```python
from build123d import *

# Parameters (mm, degrees)
F0_W     = 9
F0_H     = 9
F0_H_2   = 441
F1_DEPTH = 18
F2_DEPTH = 9


# Not quite as in the source:
# - ends of sketch curves that miss each other by under 0.0002 mm in the source are joined


with BuildPart() as f1:
    # F0 (on Front) → F1 (new body)
    with BuildSketch(Plane.XZ):
        with Locations((-1095.5, 71.3756743552)):
            Rectangle(F0_W, F0_H)
        with BuildLine():
            Line((0, 66.8756743552), (-1091, 66.8756743552))
            Line((-1091, 66.8756743552), (-1091, -374.1243256448))
            Line((-1091, -374.1243256448), (-1055, -374.1243256448))
            ThreePointArc((-1055, -374.1243256448), (-1054.8038113281, -374.1191399972), (-1054.6076226562, -374.1243256448))
            Line((-1054.6076226562, -374.1243256448), (-973.3476458471, -374.1243256448))
            Line((-973.3476458471, -374.1243256448), (0, -374.1243256448))
            Line((0, -374.1243256448), (973.3476458471, -374.1243256448))
            Line((973.3476458471, -374.1243256448), (1054.6076226562, -374.1243256448))
            ThreePointArc((1054.6076226562, -374.1243256448), (1054.8038113281, -374.1191399972), (1055, -374.1243256448))
            Line((1055, -374.1243256448), (1091, -374.1243256448))
            Line((1091, -374.1243256448), (1091, -365.1243256448))
            Line((1091, -365.1243256448), (1091, -365.0378882885))
            Line((1091, -365.0378882885), (1091, 66.8756743552))
            Line((1091, 66.8756743552), (0, 66.8756743552))
        make_face()
        with BuildLine():
            Line((-1050, -320.6243256448), (-1050, 22.3756743552))
            ThreePointArc((-1050, 22.3756743552), (-1052.4748737342, 28.3505480894), (-1046.5, 25.8756743552))
            Line((-1046.5, 25.8756743552), (0, 25.8756743552))
            Line((0, 25.8756743552), (1046.5, 25.8756743552))
            ThreePointArc((1046.5, 25.8756743552), (1052.4748737342, 28.3505480894), (1050, 22.3756743552))
            Line((1050, 22.3756743552), (1050, -320.6243256448))
            ThreePointArc((1050, -320.6243256448), (1052.4748737342, -326.5991993789), (1046.5, -324.1243256448))
            Line((1046.5, -324.1243256448), (900, -324.1243256448))
            Line((900, -324.1243256448), (900, -338.6243256448))
            ThreePointArc((900, -338.6243256448), (902.4748737342, -344.5991993789), (896.5, -342.1243256448))
            Line((896.5, -342.1243256448), (753.5000238419, -342.1243256448))
            ThreePointArc((753.5000238419, -342.1243256448), (747.5251501077, -344.5991993789), (750.0000238419, -338.6243256448))
            Line((750.0000238419, -338.6243256448), (750.0000238419, -324.1243256448))
            Line((750.0000238419, -324.1243256448), (600.0000238419, -324.1243256448))
            Line((600.0000238419, -324.1243256448), (600, -338.6243256448))
            ThreePointArc((600, -338.6243256448), (602.4748737342, -344.5991993789), (596.5, -342.1243256448))
            Line((596.5, -342.1243256448), (453.5000238419, -342.1243256448))
            ThreePointArc((453.5000238419, -342.1243256448), (447.5251501077, -344.5991993789), (450.0000238419, -338.6243256448))
            Line((450.0000238419, -338.6243256448), (450.0000238419, -324.1243256448))
            Line((450.0000238419, -324.1243256448), (300.0000238419, -324.1243256448))
            Line((300.0000238419, -324.1243256448), (300, -338.6243256448))
            ThreePointArc((300, -338.6243256448), (302.4748737342, -344.5991993789), (296.5, -342.1243256448))
            Line((296.5, -342.1243256448), (153.5000238419, -342.1243256448))
            ThreePointArc((153.5000238419, -342.1243256448), (147.5251501077, -344.5991993789), (150.0000238419, -338.6243256448))
            Line((150.0000238419, -338.6243256448), (150.0000238419, -324.1243256448))
            Line((150.0000238419, -324.1243256448), (2.38419e-05, -324.1243256448))
            Line((2.38419e-05, -324.1243256448), (-150.0000238419, -324.1243256448))
            Line((-150.0000238419, -324.1243256448), (-150.0000238419, -338.6243256448))
            ThreePointArc((-150.0000238419, -338.6243256448), (-147.5251501077, -344.5991993789), (-153.5000238419, -342.1243256448))
            Line((-153.5000238419, -342.1243256448), (-296.5, -342.1243256448))
            ThreePointArc((-296.5, -342.1243256448), (-302.4748737342, -344.5991993789), (-300, -338.6243256448))
            Line((-300, -338.6243256448), (-300, -324.1243256448))
            Line((-300, -324.1243256448), (-450.0000238419, -324.1243256448))
            Line((-450.0000238419, -324.1243256448), (-450.0000238419, -338.6243256448))
            ThreePointArc((-450.0000238419, -338.6243256448), (-447.5251501077, -344.5991993789), (-453.5000238419, -342.1243256448))
            Line((-453.5000238419, -342.1243256448), (-596.5, -342.1243256448))
            ThreePointArc((-596.5, -342.1243256448), (-602.4748737342, -344.5991993789), (-600, -338.6243256448))
            Line((-600, -338.6243256448), (-600, -324.1243256448))
            Line((-600, -324.1243256448), (-750.0000238419, -324.1243256448))
            Line((-750.0000238419, -324.1243256448), (-750.0000238419, -338.6243256448))
            ThreePointArc((-750.0000238419, -338.6243256448), (-747.5251501077, -344.5991993789), (-753.5000238419, -342.1243256448))
            Line((-753.5000238419, -342.1243256448), (-896.5, -342.1243256448))
            ThreePointArc((-896.5, -342.1243256448), (-902.4748737342, -344.5991993789), (-900, -338.6243256448))
            Line((-900, -338.6243256448), (-900, -324.1243256448))
            Line((-900, -324.1243256448), (-1046.5, -324.1243256448))
            ThreePointArc((-1046.5, -324.1243256448), (-1052.4748737342, -326.5991993789), (-1050, -320.6243256448))
        make_face(mode=Mode.SUBTRACT)
        with BuildLine():
            Line((-973.3476458471, -374.1243256448), (-1054.6076226562, -374.1243256448))
            ThreePointArc((-1054.6076226562, -374.1243256448), (-1051.7483407187, -375.721921149), (-1051.265639742, -378.9614896944))
            Line((-1051.265639742, -378.9614896944), (-1098.3606008427, -558.954299013))
            ThreePointArc((-1098.3606008427, -558.954299013), (-1097.4812264988, -563.2754093644), (-1093.523436793, -565.219938755))
            Line((-1093.523436793, -565.219938755), (-1078.8076104242, -565.219938755))
            ThreePointArc((-1078.8076104242, -565.219938755), (-1076.2129629213, -564.4940239596), (-1074.371712623, -562.5270604893))
            Line((-1074.371712623, -562.5270604893), (-977.7835436484, -376.8172039105))
            ThreePointArc((-977.7835436484, -376.8172039105), (-975.94229335, -374.8502404402), (-973.3476458471, -374.1243256448))
        make_face()
        Polygon((1100, 66.8756743552), (1091, 66.8756743552), (1091, -365.0378882885), (1091, -365.1243256448), (1091, -374.1243256448), (1100, -374.1243256448), align=None)
        Polygon((0, 75.8756743552), (-1091, 75.8756743552), (-1091, 66.8756743552), (0, 66.8756743552), (1091, 66.8756743552), (1091, 75.8756743552), align=None)
        with Locations((-1095.5, -153.6243256448)):
            Rectangle(F0_W, F0_H_2)
        with Locations((1095.5, 71.3756743552)):
            Rectangle(F0_W, F0_H)
        with BuildLine():
            Line((1054.6076226562, -374.1243256448), (973.3476458471, -374.1243256448))
            ThreePointArc((973.3476458471, -374.1243256448), (975.94229335, -374.8502404402), (977.7835436484, -376.8172039105))
            Line((977.7835436484, -376.8172039105), (1074.371712623, -562.5270604893))
            ThreePointArc((1074.371712623, -562.5270604893), (1076.2129629213, -564.4940239596), (1078.8076104242, -565.219938755))
            Line((1078.8076104242, -565.219938755), (1093.523436793, -565.219938755))
            ThreePointArc((1093.523436793, -565.219938755), (1097.4812264988, -563.2754093644), (1098.3606008427, -558.954299013))
            Line((1098.3606008427, -558.954299013), (1051.265639742, -378.9614896944))
            ThreePointArc((1051.265639742, -378.9614896944), (1051.7483407187, -375.721921149), (1054.6076226562, -374.1243256448))
        make_face()
    extrude(amount=F1_DEPTH)

    # F0 (on Front) → F2 (cut)
    with BuildSketch(Plane.XZ):
        Polygon((0, 75.8756743552), (-1091, 75.8756743552), (-1091, 66.8756743552), (0, 66.8756743552), (1091, 66.8756743552), (1091, 75.8756743552), align=None)
        with Locations((1095.5, 71.3756743552)):
            Rectangle(F0_W, F0_H)
        with Locations((-1095.5, -153.6243256448)):
            Rectangle(F0_W, F0_H_2)
        with Locations((-1095.5, 71.3756743552)):
            Rectangle(F0_W, F0_H)
        Polygon((1100, 66.8756743552), (1091, 66.8756743552), (1091, -365.0378882885), (1091, -365.1243256448), (1091, -374.1243256448), (1100, -374.1243256448), align=None)
    extrude(amount=F2_DEPTH, mode=Mode.SUBTRACT)


solid = f1.part
```
Here's how the part is built. I have some questions about the finished solid (model axes, mm). A direction names the side the tool comes from. Give positions to 0.01 mm unless a question says otherwise; leave off trailing zeros. Write each loop counter-clockwise with the first axis right and the second up, starting at its lowest first coordinate (ties: lowest second). Pieces come first, ordered by that corner, then holes. Notation, with made-up numbers: M 69.25,-37 L 73.25,-37 A12 ccw 73.25,-14 Z; hole C 42.5,55 d6. An arc over 180 degrees is marked long. Put each result on its own line as item: value. Start each with the question number.
Item 1: Thinking about a two-plate mould opening in Z: for faces 1 (the flat face through (-1026.754, -8.874, -470.972)), 2 (the flat face through (-5, 0, -341)), 3 (the flat face through (-1074.483, -8.874, -467.698)), 4 (the flat face through (1075.143, -8.874, -470.218)), which applies, +Z half, -Z half, draft (parallel to the pull), parting line (faces both ways), or undercut?
Item 2: If we section it at A-A, the plane z = -277: Write out the boundary of the cut face in (x, y), then the cut area to 3 significant figures.
Item 3: If we section it at B-B, the plane x = 194.5: Write out the boundary of the cut face in (y, z), then the cut area to 4 significant figures.
Item 4: I need wall thicknesses on L1, parallel to Z at x = 304, y = -9.5; L2, parallel to X at y = -2.5, z = 5; L3, parallel to Z at x = -433, y = -3. Which ranges of each line are inside material? Lowest first, please. Write a range as from..to.
Item 5: Will these pins go through, and if not, where does the flat tip stop? pin 1 (4 mm diameter, centred on x = 810.5, y = -6, fed in from -Z); pin 2 (11 mm diameter, centred on x = 300, z = -342.12, fed in from +Y); pin 3 (2 mm diameter, centred on y = -7.5, z = -250, fed in from +X).
Item 6: On a 3-axis mill with a long thin cutter (end or side, diameter ignored), from which of +Z, -Z, +X, -X, +Y, -Y can I reach the whole of each face in a straight line? I mean faces 5 (the flat face through (-5, -18, -338)), 6 (the flat face through (1025.4, -8.87, -468.37)). Say none if no direction works.
Values:
1. face 1: -Z half
1. face 2: draft
1. face 3: undercut
1. face 4: undercut
2. outline: M -1100,-18 L -1050,-18 L -1050,0 L -1091,0 L -1091,-9 L -1100,-9 Z; M 1050,-18 L 1100,-18 L 1100,-9 L 1091,-9 L 1091,0 L 1050,0 Z
2. area: 1,640 mm²
3. outline: M -18,-374.12 L 0,-374.12 L 0,-342.12 L -18,-342.12 Z; M -18,25.88 L 0,25.88 L 0,66.88 L -9,66.88 L -9,75.88 L -18,75.88 Z
3. area: 1,395 mm²
4. L1: -374.12..-324.12, 25.88..75.88
4. L2: -1091..-1050, 1050..1091
4. L3: -374.12..-324.12, 25.88..66.88
5. pin 1: z = -374.12
5. pin 2: y = 0
5. pin 3: x = 1091
6. face 5: +Z, -Z, +X, -X, -Y
6. face 6: -Z, +Y, -Y
